Source: CAD feature listing. Evaluate the final solid. Frame: model axes, mm. A direction names the side the tool comes from. Coordinates: 2 decimals unless noted, no trailing zeros. Order: outer loops, then holes, each group sorted by start corner. A loop starts at its lowest first (then second) coordinate and runs counter-clockwise, first axis right, second up.
Autodesk Fusion 360 part; units mm, degrees
sketch "Skizze1" plane through (0, 0, 0) normal (0, 0, 1) x (1, 0, 0) in component "Montagewinkel"
  line L0 (0, 0) -> (92, 0)
  line L1 (92, 0) -> (92, 55)
  line L2 (92, 55) -> (0, 55)
  line L3 (0, 55) -> (0, 0)
  line L4 (2, 2) -> (90, 2)
  line L5 (90, 2) -> (90, 53)
  line L6 (90, 53) -> (2, 53)
  line L7 (2, 53) -> (2, 2)
  line L8 (2, 53) -> (2, 55)
  line L9 (90, 53) -> (90, 55)
  line L10 (2, 2) -> (2, 0)
  line L11 (90, 2) -> (90, 0)
  circle A0 centre (23.5, 27.5) radius 14.5
  circle A1 centre (74.5, 22) radius 6
  circle A2 centre (74.5, 45) radius 4
  line L12 (38, 47) -> (38, 7) construction
  line L13 (68.5, 47) -> (68.5, 7) construction
  line L14 (68.5, 27.5) -> (38, 27.5) construction
  line L15 (57.25, 19.5) -> (49.25, 19.5)
  line L16 (49.25, 19.5) -> (49.25, 35.5)
  line L17 (49.25, 35.5) -> (57.25, 35.5)
  line L18 (57.25, 35.5) -> (57.25, 19.5)
  line L19 (57.25, 19.5) -> (49.25, 35.5) construction
  line L20 (49.25, 19.5) -> (57.25, 35.5) construction
  line L21 (58.85, 17.9) -> (47.65, 17.9)
  line L22 (47.65, 17.9) -> (47.65, 37.1)
  line L23 (47.65, 37.1) -> (58.85, 37.1)
  line L24 (58.85, 37.1) -> (58.85, 17.9)
  point P0 (53.25, 27.5)
  dimension "d1" = 92
  dimension "d2" = 55
  dimension "d3" = -2
  dimension "d4" = 29
  dimension "d5" = 23.5
  dimension "d6" = 27.5
  dimension "d7" = 12
  dimension "d8" = 22
  dimension "d9" = 17.5
  dimension "d10" = 8
  dimension "d11" = 10
  dimension "d12" = 17.5
  dimension "d13" = 27.5
  dimension "d14" = 8
  dimension "d15" = 16
  dimension "d16" = -1.6
extrude "Extrusion1" add sketch "Skizze1" along normal blind 2 contours L4 L5 L6 L7 in component "Montagewinkel"
extrude "Extrusion3" add sketch "Skizze1" along normal blind 6 contours L21 L22 L23 L24 in component "Montagewinkel"
extrude "Extrusion4" add sketch "Skizze1" along normal blind 50 contours L0 L2 L3 L7 L8 L10 | L0 L1 L2 L5 L9 L11 | L2 L6 L8 L9 in component "Montagewinkel"
extrude "Extrusion5" add sketch "Skizze1" along normal blind 12 contours L0 L4 L10 L11 in component "Montagewinkel"
chamfer "Fase1" distance 52 distance2 38 2 edges at (1, 0, 50) (91, 0, 50) measured on face at (31.3333, 54.3333, 50) measured on face at (31.3333, 54.3333, 50) in component "Montagewinkel"
chamfer "Fase2" distance 2 angle 45 3 edges at (46, 0, 0) (0, 27.5, 0) (92, 27.5, 0) in component "Montagewinkel"
sketch "Skizze2" plane through (0, 55, 0) normal (0, 1, 0) x (-1, 0, 0) in component "Montagewinkel"
  line L0 (-92, 2) -> (-90, 0)
  line L1 (-90, 0) -> (-2, 0)
  line L2 (-2, 0) -> (0, 2)
  line L3 (0, 2) -> (0, 50)
  line L4 (0, 50) -> (-92, 50)
  line L5 (-92, 50) -> (-92, 2)
  line L6 (0, 12) -> (-2, 12)
  line L7 (-2, 12) -> (-90, 12)
  line L8 (-90, 12) -> (-92, 12)
  line L9 (-2, 2) -> (-2, 50)
  line L10 (-90, 2) -> (-90, 50)
  circle A0 centre (-80, 19) radius 1.8
  circle A1 centre (-63, 19) radius 1.8
  circle A2 centre (-80, 31) radius 1.8
  circle A3 centre (-63, 31) radius 1.8
  circle A4 centre (-46, 19) radius 1.8
  circle A5 centre (-29, 19) radius 1.8
  circle A6 centre (-12, 19) radius 1.8
  circle A7 centre (-46, 31) radius 1.8
  circle A8 centre (-29, 31) radius 1.8
  circle A9 centre (-12, 31) radius 1.8
  circle A10 centre (-80, 43) radius 1.8
  circle A11 centre (-63, 43) radius 1.8
  circle A12 centre (-46, 43) radius 1.8
  circle A13 centre (-29, 43) radius 1.8
  circle A14 centre (-12, 43) radius 1.8
  dimension "d30" = 3.6
  dimension "d31" = 10
  dimension "d32" = 7
  dimension "d36" = 68
  dimension "d37" = 24
extrude "Extrusion6" cut sketch "Skizze2" against normal blind 2 contours A0 | A1 | A2 | A3 | A4 | A5 | A6 | A7 | A8 | A9 | A10 | A11 | A12 | A13 | A14 in component "Montagewinkel"
component "Montagewinkel" placed x (1, 0, 0) y (0, 1, 0) z (0, 0, 1) at (0, 0, 0)
equation "d5 = ( 37 / 2 ) * 1 mm + 5 mm"
equation "d6 = ( 55 / 2 ) * 1 mm"
equation "d8 = 5 mm + ( 34 / 2 ) * 1 mm"
equation "d9 = 5 mm + ( 25 / 2 ) * 1 mm"
equation "d11 = 5 mm + 5 mm"
equation "d13 = ( 55 / 2 ) * 1 mm"
1. Access query for faces 5 (the face through (91, 28, 1)), 6 (the face through (49.25, 27, 3)). Directions: +Z, -Z, +X, -X, +Y, -Y. A direction counts if a zero-diameter tool reaches every point of the face in a straight line with its end or side. Return the directions, or none.
Findings:
face 5: -Z, +X, +Y, -Y
face 6: +Z, -Z
2. Section query C-C on x = 74.5. Return loops of the section in (y, z).
Findings:
outline: (0, 2) - (2, 0) - (16, 0) - (16, 2) - (2, 2) - (2, 12) - (0, 12) - close; (28, 0) - (41, 0) - (41, 2) - (28, 2) - close; (49, 0) - (55, 0) - (55, 50) - (53, 50) - (53, 2) - (49, 2) - close
3. Section query A-A on x = 63. Return loops of the section in (y, z).
Findings:
outline: (0, 2) - (2, 0) - (55, 0) - (55, 17.2) - (53, 17.2) - (53, 2) - (2, 2) - (2, 12) - (0, 12) - close; (53, 20.8) - (55, 20.8) - (55, 29.2) - (53, 29.2) - close; (53, 32.8) - (55, 32.8) - (55, 41.2) - (53, 41.2) - close; (53, 44.8) - (55, 44.8) - (55, 50) - (53, 50) - close
4. Pin query (flat end, axial travel): P1, Ø3, axis at x = 29, z = 19, coming from the -Y side; P2, Ø4, axis at x = 29, z = 31, coming from the -Y side; P3, Ø14, axis at x = 74.5, y = 22, coming from the +Z side; P4, Ø1.5, axis at x = 48.5, y = 18.5, coming from the +Z side. Return the tip coordinate at first contact, or that it passes through.
Findings:
P1: passes through
P2: stops at y = 53
P3: stops at z = 2
P4: stops at z = 6
5. Section query B-B on x = 23.5. Return loops of the section in (y, z), plus the area to 3 significant figures.
Findings:
outline: (0, 2) - (2, 0) - (13, 0) - (13, 2) - (2, 2) - (2, 12) - (0, 12) - close; (42, 0) - (55, 0) - (55, 50) - (53, 50) - (53, 2) - (42, 2) - close
area: 166 mm2
6. Draft query along Y for faces 1 (the face through (58.85, 28, 4)), 2 (the face through (27.283, 54.014, 31.541)), 3 (the face through (1, 26, 31)), 4 (the face through (53, 17.9, 4)). Return one class per face: released by +Y, released by -Y, zero draft, split by the parting line, or undercut.
Findings:
face 1: undercut
face 2: zero draft
face 3: released by -Y
face 4: undercut
7. Section query D-D on y = 30.5. Return loops of the section in (x, z).
Findings:
outline: (0, 2) - (2, 0) - (9.31, 0) - (9.31, 2) - (2, 2) - (2, 34.29) - (0, 34.29) - close; (37.69, 0) - (49.25, 0) - (49.25, 6) - (47.65, 6) - (47.65, 2) - (37.69, 2) - close; (57.25, 0) - (90, 0) - (92, 2) - (92, 34.29) - (90, 34.29) - (90, 2) - (58.85, 2) - (58.85, 6) - (57.25, 6) - close
8. Ray query, line 1 (X direction, y = 22, z = 3.5); line 2 (Z direction, x = 80, y = 54.2); line 3 (X direction, y = 31.5, z = 30). Return the intervals inside material, ascending.
Findings:
line 1: x = 0 to 2, 47.65 to 49.25, 57.25 to 58.85, 90 to 92
line 2: z = 0 to 17.2, 20.8 to 29.2, 32.8 to 41.2, 44.8 to 50
line 3: x = 0 to 2, 90 to 92
